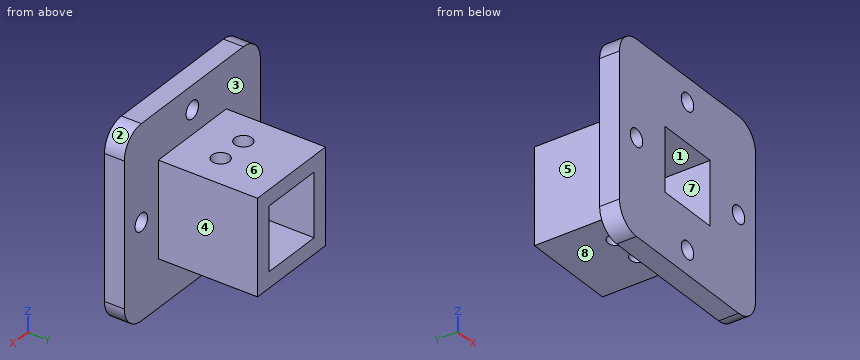
from build123d import *

# Parameters (mm, degrees)
SKETCH_1_W          = 24
SKETCH_1_H          = 24
SKETCH_1_W_2        = 16
SKETCH_1_H_2        = 16
EXTRUDE_1_DEPTH     = 30
SKETCH_2_R          = 2.2
CUT_EXTRUDE_1_DEPTH = 31
SKETCH_3_W          = 6
SKETCH_3_H          = 6
SKETCH_3_W_2        = 24
SKETCH_3_H_2        = 24
EXTRUDE_3_DEPTH     = 5
FILLET_1_R          = 6
SKETCH_4_R          = 2.2
CUT_EXTRUDE_2_DEPTH = 5


with BuildPart() as part:
    # 草图1 → 凸台-拉伸1 (new body)
    with BuildSketch(Plane(origin=(0, 0, 0), x_dir=(1, 0, 0), z_dir=(0, 1, 0))):
        with Locations((12, 12)):
            Rectangle(SKETCH_1_W, SKETCH_1_H)
        with Locations((12, 12)):
            Rectangle(SKETCH_1_W_2, SKETCH_1_H_2, mode=Mode.SUBTRACT)
    extrude(amount=EXTRUDE_1_DEPTH)

    # 草图2 → 切除-拉伸1 (cut)
    with BuildSketch(Plane.XY):
        with Locations(Location((8, 15, 0), (0, 0, 180))):
            Circle(SKETCH_2_R)
        with Locations(Location((16, 15, 0), (0, 0, 180))):
            Circle(SKETCH_2_R)
    extrude(amount=-CUT_EXTRUDE_1_DEPTH, mode=Mode.SUBTRACT)

    # 草图3 → 凸台-拉伸3 (add)
    # profile 1 of 5: a face of its own
    with BuildSketch(Plane.XZ):
        with Locations((-9, -33)):
            Rectangle(SKETCH_3_W, SKETCH_3_H)
    # profile 2 of 5: a face of its own
    with BuildSketch(Plane.XZ):
        Polygon((-12, -30), (-6, -30), (-6, 6), (0, 6), (30, 6), (30, 12), (-12, 12), align=None)
    # profile 3 of 5: a face of its own
    with BuildSketch(Plane.XZ):
        Polygon((30, -30), (30, 6), (0, 6), (-6, 6), (-6, -30), align=None)
        with Locations((12, -12)):
            Rectangle(SKETCH_3_W_2, SKETCH_3_H_2, mode=Mode.SUBTRACT)
    # profile 4 of 5: a face of its own
    with BuildSketch(Plane.XZ):
        Polygon((30, -30), (-6, -30), (-6, -36), (36, -36), (36, 6), (30, 6), align=None)
    # profile 5 of 5: a face of its own
    with BuildSketch(Plane.XZ):
        with Locations((33, 9)):
            Rectangle(SKETCH_3_W, SKETCH_3_H)
    extrude(amount=-EXTRUDE_3_DEPTH)

    # 圆角1
    fillet_1_edges = [part.edges().sort_by_distance(p)[0] for p in [
        (36, 2.5, 12),
        (36, 2.5, -36),
        (-12, 2.5, -36),
        (-12, 2.5, 12),
    ]]
    fillet(fillet_1_edges, radius=FILLET_1_R)

    # 草图4 → 切除-拉伸2 (cut)
    with BuildSketch(Plane(origin=(0, 5, 0), x_dir=(1, 0, 0), z_dir=(0, 1, 0))):
        with Locations(Location((12, -6, 0), (0, 0, 270))):
            Circle(SKETCH_4_R)
        with Locations(Location((-6, 12, 0), (0, 0, 270))):
            Circle(SKETCH_4_R)
        with Locations(Location((12, 30, 0), (0, 0, 270))):
            Circle(SKETCH_4_R)
        with Locations(Location((30, 12, 0), (0, 0, 270))):
            Circle(SKETCH_4_R)
    extrude(amount=-CUT_EXTRUDE_2_DEPTH, mode=Mode.SUBTRACT)


solid = part.part
CAD build for the part. Positions are in the model's coordinates, mm. Face numbers are marked on the shaded views. A direction names the side the tool comes from. Round coordinates to 2 decimals unless told otherwise and drop trailing zeros. Loops run counter-clockwise (first coordinate to the right, second up) from the corner with the lowest first, then second, coordinate; pieces in that order, holes last. Notation, with made-up numbers: (6, 77.25) - (54, 77.25) arc R27 cw to (54, 95.25) - close; hole circle Ø5 at (25, 36). An arc over 180 degrees is marked (long way). Put each result on its own line as item: value.
1. Two-plate mould, pull along X, no slides. Class the marked faces 1, 2 and 3: released by +X, released by -X, zero draft, split by the parting line, or undercut.
Geometry check:
face 1: undercut
face 2: released by +X
face 3: zero draft
2. Wall check: line 1 (X direction, y = 2.8, z = -12); line 2 (X direction, y = 15, z = -2.9); line 3 (Z direction, x = 10, y = 21.75). Give the ranges that are in metal, low to high.
Geometry check:
line 1: -12 to -8.2, -3.8 to 4, 20 to 27.8, 32.2 to 36
line 2: 0 to 5.8, 10.2 to 13.8, 18.2 to 24
line 3: -24 to -20, -4 to 0
3. Slice it at C-C on y = 11.5. List the corners of the cut face in (x, z).
Geometry check:
outline: (0, -24) - (24, -24) - (24, 0) - (0, 0) - close; hole (4, -20) - (20, -20) - (20, -4) - (4, -4) - close
4. Slice it at A-A on z = -12. List the corners of the cut face in (x, y), and give its area (3 significant figures).
Geometry check:
outline: (-12, 0) - (-8.2, 0) - (-8.2, 5) - (-12, 5) - close; (-3.8, 0) - (4, 0) - (4, 30) - (0, 30) - (0, 5) - (-3.8, 5) - close; (20, 0) - (27.8, 0) - (27.8, 5) - (24, 5) - (24, 30) - (20, 30) - close; (32.2, 0) - (36, 0) - (36, 5) - (32.2, 5) - close
area: 316 mm²
5. Pin check, flat tips, straight feed: P1, Ø17.5, axis at y = 19, z = -10, coming from the -X side; P2, Ø10, axis at x = 30.5, z = -23, coming from the -Y side; P3, Ø7, axis at y = 22, z = -7, coming from the +X side; P4, Ø3.5, axis at x = -6, z = -12, coming from the +Y side. Stop position of each tip, or through.
Geometry check:
P1: x = 0
P2: y = 0
P3: x = 24
P4: through
6. Slice it at B-B on x = 16. List the corners of the cut face in (y, z).
Geometry check:
outline: (0, -36) - (5, -36) - (5, -24) - (12.8, -24) - (12.8, -20) - (0, -20) - close; (0, -4) - (12.8, -4) - (12.8, 0) - (5, 0) - (5, 12) - (0, 12) - close; (17.2, -24) - (30, -24) - (30, -20) - (17.2, -20) - close; (17.2, -4) - (30, -4) - (30, 0) - (17.2, 0) - close
7. 3-axis set-ups, long thin cutter, end or side, ignore diameter. For the marked faces 4, 5, 6, 7 and 8: which of +Z, -Z, +X, -X, +Y, -Y reach the whole face in a straight line?
Geometry check:
face 4: +Z, -Z, +X, +Y
face 5: +Z, -Z, -X, +Y
face 6: +Z, +X, -X, +Y
face 7: +Y, -Y
face 8: -Z, +X, -X, +Y
8. Slice it at D-D on y = 16.25. List the corners of the cut face in (x, z), and give its area (3 significant figures).
Geometry check:
outline: (0, -24) - (6.19, -24) - (6.19, -20) - (4, -20) - (4, -4) - (6.19, -4) - (6.19, 0) - (0, 0) - close; (9.81, -24) - (14.19, -24) - (14.19, -20) - (9.81, -20) - close; (9.81, -4) - (14.19, -4) - (14.19, 0) - (9.81, 0) - close; (17.81, -24) - (24, -24) - (24, 0) - (17.81, 0) - (17.81, -4) - (20, -4) - (20, -20) - (17.81, -20) - close
area: 262 mm²
